Print and shaded views of the part. All mm, measured from the part's lowest x, y and z. Coordinates: 2 decimals unless noted, no trailing zeros. Loops run counter-clockwise (first coordinate to the right, second up) from the corner with the lowest first, then second, coordinate; pieces in that order, holes last.
1) Saw through at B-B, the plane y = 2.3. Give the number of separate pieces and of enclosed holes in the cut face, and give its area (3 significant figures).
2) Saw through at C-C, the plane x = 187. Write the cut outline in (y, z) (1 decimal), and give its area (3 significant figures).
3) Wall check: line 1 along X through (y, z) = (0.6, 37.5); line 2 along Z through (x, y) = (85, 0.75); line 3 along Z through (x, y) = (184.5, 0.65) (1 decimal). Give the ranges that are in metal, low to high.
4) Pin check, flat tip, straight feed: pin 1 Ø1.6 at (y, z) = (1, 56) entering from -X. Stop position of the tip, or through.
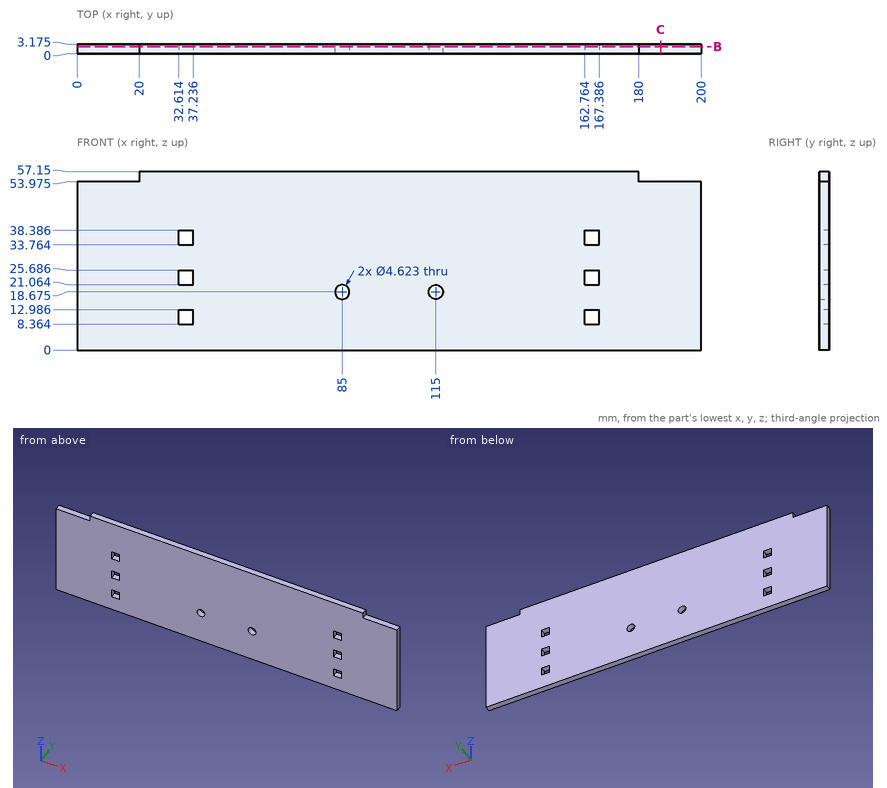
Data:
1. separate pieces: 1
1. enclosed holes: 8
1. area: 11,100 mm2
2. outline: (0, 0) - (3.2, 0) - (3.2, 54) - (0, 54) - close
2. area: 171 mm2
3. line 1: x = 0 to 32.61, 37.24 to 162.76, 167.39 to 200
3. line 2: z = 0 to 16.36, 20.99 to 57.15
3. line 3: z = 0 to 54
4. pin 1: stops at x = 20
